```python
from build123d import *

# Parameters (mm, degrees)
SKETCH1_W                = 65
SKETCH1_H                = 40
BOSS_EXTRUDE1_DEPTH      = 130
SHELL1_T                 = -4
FILLET1_R                = 5
CUT_EXTRUDE1_DEPTH       = 21
CUT_EXTRUDE1_DEPTH_BACK  = 21
SKETCH3_W                = 17.5
SKETCH3_H                = 50
CUT_EXTRUDE2_DEPTH       = 21
CUT_EXTRUDE2_DEPTH_BACK  = 21
SKETCH5_W                = 2
SKETCH5_H                = 50
BOSS_EXTRUDE2_DEPTH      = 3
SKETCH6_W                = 2
SKETCH6_H                = 30
BOSS_EXTRUDE3_DEPTH      = 3
SKETCH8_W                = 70
SKETCH8_H                = 66
BOSS_EXTRUDE4_DEPTH      = 20
SKETCH10_W               = 60
SKETCH10_H               = 12
CUT_EXTRUDE4_DEPTH       = 45
SKETCH23_W               = 2
SKETCH23_H               = 15
CUT_EXTRUDE10_DEPTH      = 10
CUT_EXTRUDE11_START      = -10
SKETCH24_R               = 1.7
CUT_EXTRUDE11_DEPTH      = 13.5
SKETCH27_W               = 70
SKETCH27_H               = 33
CUT_EXTRUDE12_DEPTH      = 132.543487266
CUT_EXTRUDE12_DEPTH_BACK = 21
SKETCH31_R               = 2.7
CUT_EXTRUDE13_DEPTH      = 1
CUT_EXTRUDE13_DEPTH_BACK = 34
SKETCH34_R               = 1.7
CUT_EXTRUDE15_DEPTH      = 132.543487266
CUT_EXTRUDE15_DEPTH_BACK = 21
SKETCH37_W               = 6
SKETCH37_H               = 6
CUT_EXTRUDE17_DEPTH      = 3.5
CUT_EXTRUDE17_DEPTH_BACK = 68.5
SKETCH38_W               = 15
SKETCH38_H               = 17
BOSS_EXTRUDE9_DEPTH      = 2.5
SKETCH41_R               = 4
CUT_EXTRUDE18_DEPTH      = 2.4
SKETCH42_W               = 4.6
SKETCH42_H               = 4
BOSS_EXTRUDE10_DEPTH     = 3
CUT_EXTRUDE19_DEPTH      = 5
FILLET2_R                = 1
SKETCH46_R               = 1.7
CUT_EXTRUDE20_DEPTH      = 10
SKETCH50_W               = 15
SKETCH50_H               = 15
BOSS_EXTRUDE11_DEPTH     = 16
SKETCH51_R               = 2.7
CUT_EXTRUDE21_DEPTH      = 16.153953894
CUT_EXTRUDE21_DEPTH_BACK = 21


with BuildPart() as part:
    # Sketch1 → Boss-Extrude1 (new body)
    with BuildSketch(Plane(origin=(0, 0, 0), x_dir=(1, 0, 0), z_dir=(0, 1, 0))):
        Rectangle(SKETCH1_W, SKETCH1_H)
    extrude(amount=BOSS_EXTRUDE1_DEPTH)

    # Shell1
    shell1_openings = [part.faces().sort_by_distance(p)[0] for p in [
        (0, 130, 0),
        (0, 0, 0),
    ]]
    offset(amount=SHELL1_T, openings=shell1_openings, kind=Kind.INTERSECTION)

    # Fillet1
    fillet1_edges = [part.edges().sort_by_distance(p)[0] for p in [
        (32.5, 65, 20),
        (-32.5, 65, 20),
        (-32.5, 65, -20),
        (32.5, 65, -20),
    ]]
    fillet(fillet1_edges, radius=FILLET1_R)

    # Sketch2 → Cut-Extrude1 (cut, two sides)
    with BuildSketch(Plane.XY) as cut_extrude1_sk:
        Polygon((-5.5, 130), (-32.5, 85), (-32.5, 130), align=None)
    extrude(amount=CUT_EXTRUDE1_DEPTH, mode=Mode.SUBTRACT)
    extrude(cut_extrude1_sk.sketch, amount=-CUT_EXTRUDE1_DEPTH_BACK, mode=Mode.SUBTRACT)

    # Sketch3 → Cut-Extrude2 (cut, two sides)
    with BuildSketch(Plane.XY) as cut_extrude2_sk:
        with Locations((23.75, 105)):
            Rectangle(SKETCH3_W, SKETCH3_H)
    extrude(amount=CUT_EXTRUDE2_DEPTH, mode=Mode.SUBTRACT)
    extrude(cut_extrude2_sk.sketch, amount=-CUT_EXTRUDE2_DEPTH_BACK, mode=Mode.SUBTRACT)

    # Sketch5 → Boss-Extrude2 (add)
    with BuildSketch(Plane(origin=(15, 0, 0), x_dir=(0, 0, -1), z_dir=(1, 0, 0))):
        with Locations((-18, 105)):
            Rectangle(SKETCH5_W, SKETCH5_H)
    boss_extrude2 = extrude(amount=BOSS_EXTRUDE2_DEPTH)

    # Mirror1: Boss-Extrude2 across plane
    add(boss_extrude2.mirror(Plane.XY))

    # Sketch6 → Boss-Extrude3 (add)
    with BuildSketch(Plane(origin=(-61.397058824, 36.838235294, 0), x_dir=(0, 0, 1), z_dir=(-0.857492926, 0.514495755, 0))):
        with Locations((-18, 93.644353688)):
            Rectangle(SKETCH6_W, SKETCH6_H)
    boss_extrude3 = extrude(amount=BOSS_EXTRUDE3_DEPTH)

    # Mirror2: Boss-Extrude3 across plane
    add(boss_extrude3.mirror(Plane.XY))

    # Sketch8 → Boss-Extrude4 (add)
    with BuildSketch(Plane(origin=(0, 0, 0), x_dir=(1, 0, 0), z_dir=(0, 1, 0))):
        Rectangle(SKETCH8_W, SKETCH8_H)
    extrude(amount=-BOSS_EXTRUDE4_DEPTH)

    # Sketch10 → Cut-Extrude4 (cut)
    with BuildSketch(Plane.ZY.offset(35)):
        with Locations((0, -10)):
            Rectangle(SKETCH10_W, SKETCH10_H)
    extrude(amount=-CUT_EXTRUDE4_DEPTH, mode=Mode.SUBTRACT)

    # Sketch23 → Cut-Extrude10 (cut)
    with BuildSketch(Plane(origin=(0, 80, 0), x_dir=(1, 0, 0), z_dir=(0, 1, 0))):
        with Locations((30.5, 0)):
            Rectangle(SKETCH23_W, SKETCH23_H)
    extrude(amount=-CUT_EXTRUDE10_DEPTH, mode=Mode.SUBTRACT)

    # Sketch24 → Cut-Extrude11 (cut)
    with BuildSketch(Plane(origin=(32.5, 0, 0), x_dir=(0, 0, -1), z_dir=(1, 0, 0)).offset(CUT_EXTRUDE11_START)):
        with Locations((-4, 76)):
            Circle(SKETCH24_R)
    cut_extrude11 = extrude(amount=CUT_EXTRUDE11_DEPTH, mode=Mode.SUBTRACT)

    # Mirror4: Cut-Extrude11 across plane
    add(cut_extrude11.mirror(Plane.XY), mode=Mode.SUBTRACT)

    # Sketch27 → Cut-Extrude12 (cut, two sides)
    with BuildSketch(Plane(origin=(0, 0, 0), x_dir=(1, 0, 0), z_dir=(0, 1, 0))) as cut_extrude12_sk:
        with Locations((0, 16.5)):
            Rectangle(SKETCH27_W, SKETCH27_H)
    extrude(amount=CUT_EXTRUDE12_DEPTH, mode=Mode.SUBTRACT)
    extrude(cut_extrude12_sk.sketch, amount=-CUT_EXTRUDE12_DEPTH_BACK, mode=Mode.SUBTRACT)

    # Sketch31 → Cut-Extrude13 (cut, two sides)
    with BuildSketch(Plane.XY.offset(33)) as cut_extrude13_sk:
        with Locations((27, -11)):
            Circle(SKETCH31_R)
    extrude(amount=CUT_EXTRUDE13_DEPTH, mode=Mode.SUBTRACT)
    extrude(cut_extrude13_sk.sketch, amount=-CUT_EXTRUDE13_DEPTH_BACK, mode=Mode.SUBTRACT)

    # Sketch34 → Cut-Extrude15 (cut, two sides)
    with BuildSketch(Plane(origin=(0, 0, 0), x_dir=(1, 0, 0), z_dir=(0, 1, 0))) as cut_extrude15_sk:
        with Locations((0, -27)):
            Circle(SKETCH34_R)
    extrude(amount=CUT_EXTRUDE15_DEPTH, mode=Mode.SUBTRACT)
    extrude(cut_extrude15_sk.sketch, amount=-CUT_EXTRUDE15_DEPTH_BACK, mode=Mode.SUBTRACT)

    # Sketch37 → Cut-Extrude17 (cut, two sides)
    with BuildSketch(Plane(origin=(32.5, 0, 0), x_dir=(0, 0, -1), z_dir=(1, 0, 0))) as cut_extrude17_sk:
        with Locations((-3, 20)):
            Rectangle(SKETCH37_W, SKETCH37_H)
    extrude(amount=CUT_EXTRUDE17_DEPTH, mode=Mode.SUBTRACT)
    extrude(cut_extrude17_sk.sketch, amount=-CUT_EXTRUDE17_DEPTH_BACK, mode=Mode.SUBTRACT)

    # Sketch38 → Boss-Extrude9 (add)
    with BuildSketch(Plane(origin=(32.5, 0, 0), x_dir=(0, 0, -1), z_dir=(1, 0, 0))):
        with Locations((-7.5, 8.5)):
            Rectangle(SKETCH38_W, SKETCH38_H)
    extrude(amount=BOSS_EXTRUDE9_DEPTH)

    # Sketch41 → Cut-Extrude18 (cut)
    with BuildSketch(Plane(origin=(0, -20, 0), x_dir=(-1, 0, 0), z_dir=(0, -1, 0))):
        with Locations((0, -27)):
            Circle(SKETCH41_R)
    extrude(amount=-CUT_EXTRUDE18_DEPTH, mode=Mode.SUBTRACT)

    # Sketch42 → Boss-Extrude10 (add)
    with BuildSketch(Plane.XY.offset(33)):
        with Locations((-27.1, -18)):
            Rectangle(SKETCH42_W, SKETCH42_H)
    extrude(amount=BOSS_EXTRUDE10_DEPTH)

    # Sketch43 → Cut-Extrude19 (cut, through all)
    with BuildSketch(Plane(origin=(0, -16, 0), x_dir=(1, 0, 0), z_dir=(0, 1, 0))):
        Polygon((-24.8, -36), (-29.4, -33), (-29.4, -36), align=None)
    extrude(amount=-CUT_EXTRUDE19_DEPTH, mode=Mode.SUBTRACT)

    # Fillet2
    fillet2_edges = [part.edges().sort_by_distance(p)[0] for p in [
        (-24.8, -18, 36),
    ]]
    fillet(fillet2_edges, radius=FILLET2_R)

    # Sketch46 → Cut-Extrude20 (cut)
    with BuildSketch(Plane.XY.offset(20)):
        with Locations((-6.357492926, 118.852591966)):
            Circle(SKETCH46_R)
    extrude(amount=-CUT_EXTRUDE20_DEPTH, mode=Mode.SUBTRACT)

    # Sketch50 → Boss-Extrude11 (add)
    with BuildSketch(Plane(origin=(0, 0, 16), x_dir=(-1, 0, 0), z_dir=(0, 0, -1))):
        with Locations((21, 7.5)):
            Rectangle(SKETCH50_W, SKETCH50_H)
    extrude(amount=BOSS_EXTRUDE11_DEPTH)

    # Sketch51 → Cut-Extrude21 (cut, two sides)
    with BuildSketch(Plane.XY.offset(20)) as cut_extrude21_sk:
        with Locations((-22.5, 5)):
            Circle(SKETCH51_R)
    extrude(amount=CUT_EXTRUDE21_DEPTH, mode=Mode.SUBTRACT)
    extrude(cut_extrude21_sk.sketch, amount=-CUT_EXTRUDE21_DEPTH_BACK, mode=Mode.SUBTRACT)


solid = part.part
```
Geometry check sheet. Reference: the model listing, model coordinates, mm. A direction names the side the tool comes from. Give positions to 0.01 mm unless a question says otherwise; leave off trailing zeros. Order: outer loops, then holes, each group sorted by start corner. A loop starts at its lowest first (then second) coordinate and runs counter-clockwise, first axis right, second up. Notation, with made-up numbers: (36, 10) - (90, 10) arc R12 cw to (90, 25) - close; hole circle Ø1 at (-34, 80.25). An arc over 180 degrees is marked (long way). Answer in a Markdown table with one row per item. Add a question column.
Q1. Material ranges on probe 1 along X at (y, z) = (-17.1, 27); probe 2 along X at (y, z) = (35, 12.5); probe 3 along Y at (x, z) = (-1, 5), recorded low to high. Write a range as from..to.
Q2. Mould release check, pull along X, two halves, no side actions. Record for faces 1 (the flat face through (-31, 58, 0)), 2 (the flat face through (-32.5, 42, 8)), 3 (the flat face through (31.5, 74, 4)): pulls with the +X half, pulls with the -X half, needs draft (parallel to the pull), parting line crosses it, or undercut.
Q3. Gauge pin test, flat ends, axial feed: pin 1 (4.5 mm diameter, centred on y = 76, z = 4, fed in from -X); pin 2 (16.5 mm diameter, centred on y = 40, z = 5, fed in from +X); pin 3 (5 mm diameter, centred on x = -16, z = 18.5, fed in from +Y); pin 4 (5 mm diameter, centred on y = 1.5, z = 30.5, fed in from +X). Record the tip position at first contact, or that the pin passes through.
Q4. Cross-section at B-B, the plane z = 27. Enter the section's corners in (x, y).
Q5. Cross-section at D-D, the plane z = 4. Count the separate pieces of the cut face and the enclosed holes in it, then the cut area to 3 significant figures.
Q6. Tool access check on faces 4 (the flat face through (33, 17, 6)), 5 (the flat face through (7, 0, 8)), 6 (the flat face through (-15, 118, 19)), 7 (the cylindrical face through (29, 74.5, 3.2)), 8 (the flat face through (10, -10, 15)). Record the directions out of +Z, -Z, +X, -X, +Y, -Y that give a thin tool (end or side, any length) a straight path to the whole face; none if there is none.
Q7. Cross-section at C-C, the plane y = -11. Enter the section's corners in (x, z).
Q8. Cross-section at A-A, the plane y = 76. Enter the section's corners in (x, z).
Check values:
| question | item | result |
|---|---|---|
| 1 | probe 1 | x = -35..-1.7, 1.7..35 |
| 1 | probe 2 | x = -32.5..-28.5, 28.5..32.5 |
| 1 | probe 3 | y = -20..-16, -4..0 |
| 2 | face 1 | needs draft |
| 2 | face 2 | pulls with the -X half |
| 2 | face 3 | undercut |
| 3 | pin 1 | stops at x = -32.5 |
| 3 | pin 2 | stops at x = 32.5 |
| 3 | pin 3 | stops at y = 122.5 |
| 3 | pin 4 | stops at x = 35 |
| 4 | outline | (-35, -20) - (-4, -20) - (-4, -17.6) - (-1.7, -17.6) - (-1.7, -16) - (-35, -16) - close; (-35, -4) - (-1.7, -4) - (-1.7, 0) - (-35, 0) - close; (1.7, -17.6) - (4, -17.6) - (4, -20) - (35, -20) - (35, 0) - (1.7, 0) - (1.7, -4) - (10, -4) - (10, -16) - (1.7, -16) - close; hole circle Ø5.4 at (27, -11) |
| 5 | separate pieces | 5 |
| 5 | enclosed holes | 2 |
| 5 | area | 1,680 mm^2 |
| 6 | face 4 | -Z, +X |
| 6 | face 5 | -Z, +Y |
| 6 | face 6 | +Z, -X, +Y |
| 6 | face 7 | +X |
| 6 | face 8 | -Z, -X |
| 7 | outline | (-35, 30) - (10, 30) - (10, 0) - (24.3, 0) - (24.3, 33) - (-35, 33) - close; (29.7, 0) - (35, 0) - (35, 33) - (29.7, 33) - close |
| 8 | outline | (-32.5, 0) - (-28.5, 0) - (-28.5, 16) - (28.5, 16) - (28.5, 5.7) - (29.5, 5.7) - (29.5, 7.5) - (31.5, 7.5) - (31.5, 5.7) - (32.5, 5.7) - (32.5, 15) arc R5 ccw to (27.5, 20) - (-27.5, 20) arc R5 ccw to (-32.5, 15) - close; (28.5, 0) - (29.5, 0) - (29.5, 2.3) - (28.5, 2.3) - close; (31.5, 0) - (32.5, 0) - (32.5, 2.3) - (31.5, 2.3) - close |
